CAD build for the part. Positions are in the model's coordinates, mm. A direction names the side the tool comes from. Coordinates: 2 decimals unless noted, no trailing zeros. Use one line per item in the form item = value.
```python
from build123d import *

# Parameters (mm, degrees)
F0_R     = 11.3175
F1_DEPTH = 7


with BuildPart() as f1:
    # F0 (on Top) → F1 (new body)
    with BuildSketch(Plane.XY):
        with BuildLine():
            Line((-4.290395086, 17.5929758698), (-5.0968573363, 12.6047609374))
            ThreePointArc((-5.0968573363, 12.6047609374), (-8.1126471986, 11.2557929743), (-10.6780268252, 9.1740796342))
            Line((-10.6780268252, 9.1740796342), (-26.7856623977, 15.1404356584))
            add(Edge.make_bspline(
                [(-26.7856623977, 18.2235073298), (-24.4614947587, 18.7465790659), (-17.7473041348, 19.5727238501), (-24.8232074873, 15.7483036), (-26.7856623977, 15.1404356584)],
                knots=[0, 0, 0, 0, 0.4812154975, 1, 1, 1, 1], degree=3))
            ThreePointArc((-26.7856623977, 18.2235073298), (-37.6467894522, 11.8899380245), (-41.7342770438, 0))
            ThreePointArc((-41.7342770438, 0), (-37.6467894522, -11.8899380245), (-26.7856623977, -18.2235073298))
            add(Edge.make_bspline(
                [(-26.7856623977, -18.2235073298), (-24.4614947587, -18.7465790659), (-17.7473041348, -19.5727238501), (-24.8232074873, -15.7483036), (-26.7856623977, -15.1404356584)],
                knots=[0, 0, 0, 0, 0.4812154975, 1, 1, 1, 1], degree=3))
            Line((-26.7856623977, -15.1404356584), (-10.6780268252, -9.1740796342))
            ThreePointArc((-10.6780268252, -9.1740796342), (-6.4090636856, -12.1387429064), (-1.3792073587, -13.447872363))
            Line((-1.3792073587, -13.447872363), (0, -17.6072642207))
            Line((0, -17.6072642207), (1.3792073587, -13.447872363))
            ThreePointArc((1.3792073587, -13.447872363), (6.4090636856, -12.1387429064), (10.6780268252, -9.1740796342))
            Line((10.6780268252, -9.1740796342), (26.7856623977, -15.1404356584))
            add(Edge.make_bspline(
                [(26.7856623977, -18.2235073298), (24.4614947587, -18.7465790659), (17.7473041348, -19.5727238501), (24.8232074873, -15.7483036), (26.7856623977, -15.1404356584)],
                knots=[0, 0, 0, 0, 0.4812154975, 1, 1, 1, 1], degree=3))
            ThreePointArc((26.7856623977, -18.2235073298), (37.6467894522, -11.8899380245), (41.7342770438, 0))
            ThreePointArc((41.7342770438, 0), (37.6467894522, 11.8899380245), (26.7856623977, 18.2235073298))
            add(Edge.make_bspline(
                [(26.7856623977, 18.2235073298), (24.4614947587, 18.7465790659), (17.7473041348, 19.5727238501), (24.8232074873, 15.7483036), (26.7856623977, 15.1404356584)],
                knots=[0, 0, 0, 0, 0.4812154975, 1, 1, 1, 1], degree=3))
            Line((26.7856623977, 15.1404356584), (10.6780268252, 9.1740796342))
            ThreePointArc((10.6780268252, 9.1740796342), (8.1126471986, 11.2557929743), (5.0968573363, 12.6047609374))
            Line((5.0968573363, 12.6047609374), (4.290395086, 17.5929758698))
            Line((4.290395086, 17.5929758698), (4.1471831501, 17.5929758698))
            Line((4.1471831501, 17.5929758698), (1.8972994294, 12.6047609374))
            ThreePointArc((1.8972994294, 12.6047609374), (0, 13.2116865157), (-1.8972994294, 12.6047609374))
            Line((-1.8972994294, 12.6047609374), (-4.1471831501, 17.5929758698))
            Line((-4.1471831501, 17.5929758698), (-4.290395086, 17.5929758698))
        make_face()
        with Locations((-26.7856623977, 0)):
            Circle(F0_R, mode=Mode.SUBTRACT)
        Circle(F0_R, mode=Mode.SUBTRACT)
        with Locations((26.7856623977, 0)):
            Circle(F0_R, mode=Mode.SUBTRACT)
    extrude(amount=F1_DEPTH)


solid = f1.part
```
Item 1: Cut at A-A, the plane z = 1.5. State how many separate pieces and enclosed holes the cut face has, plus the area to 3 significant figures.
Derived:
separate_pieces = 1
enclosed_holes = 3
area = 990 mm²
Item 2: Drop flat-ended pins along their axis: pin 1 (2 mm diameter, centred on x = 24.5, z = 5.5, fed in from +Y); pin 2 (20.5 mm diameter, centred on x = 26.79, y = 0, fed in from -Z); pin 3 (4 mm diameter, centred on y = -8, z = 4, fed in from -X); pin 4 (4 mm diameter, centred on y = -11, z = 2.5, fed in from +X). Give the stop position or say it passes through.
Derived:
pin_1 = 18.76
pin_2 = through
pin_3 = -40.86
pin_4 = 39.58
Item 3: Drill centre lines: line 1 (Y direction, x = -21.5, z = 1.5); line 2 (X direction, y = -5, z = 1.25); line 3 (X direction, y = 16, z = 1.5). Where is each one in solid material? Low to high. Write a range as [from, to].
Derived:
line_1 = [-18.73, -17.96], [-13.18, -10.01], [10.01, 13.18], [17.96, 18.73]
line_2 = [-41.16, -36.94], [-16.63, -10.15], [10.15, 16.63], [36.94, 41.16]
line_3 = [-32.84, -24.68], [-4.55, -3.43], [3.43, 4.55], [24.68, 32.84]
Item 4: Two-plate mould, pull along Y, no slides. Class faces 1 (the face through (-6, -10, 7)), 2 (the face through (-2.45, -11.05, 3.45)), 3 (the face through (8.2, 11.2, 3.5)), 4 (the face through (6.34, -12.17, 3.45)): +Y half, -Y half, draft (parallel to the pull), parting line (faces both ways), or undercut.
Derived:
face_1 = draft
face_2 = undercut
face_3 = +Y half
face_4 = -Y half
Item 5: 3-axis set-ups, long thin cutter, end or side, ignore diameter. For faces 5 (the face through (18.619, -12.115, 3.451)), 6 (the face through (3.038, 15.134, 3.451)), 7 (the face through (-6, -10, 0)), 8 (the face through (0.68, -15.56, 3.45)): which of +Z, -Z, +X, -X, +Y, -Y reach the whole face in a straight line?
Derived:
face_5 = +Z, -Z
face_6 = +Z, -Z, +Y
face_7 = -Z, +X, -X, +Y, -Y
face_8 = +Z, -Z, -Y
